Source: CAD feature listing. Evaluate the final solid. Frame: model axes, mm. Give positions to 0.01 mm unless a question says otherwise; leave off trailing zeros. Answer in a Markdown table with one row per item.
Autodesk Inventor part; units mm, degrees
ref_plane "YZ Plane" through (0, 0, 0) normal (1, 0, 0) x (0, 1, 0)
ref_plane "XZ Plane" through (0, 0, 0) normal (0, 1, 0) x (-1, 0, 0)
ref_plane "XY Plane" through (0, 0, 0) normal (0, 0, 1) x (1, 0, 0)
sketch "Sketch1" plane through (0, 0, 0) normal (1, 0, 0) x (0, 1, 0)
  line L0 (0, 0) -> (25.4, 0) construction
  line L1 (25.4, 0) -> (25.4, -1.5875) construction
  line L2 (25.4, -1.5875) -> (0, -1.5875) construction
  line L3 (0, -1.5875) -> (0, 0) construction
  circle A0 centre (4.7625, 3.175) radius 4.7625 construction
  line L4 (25.4, 0) -> (25.4, -1.5875)
  line L5 (25.4, -1.5875) -> (4.7625, -1.5875)
  line L6 (25.4, 0) -> (8.3123, 0)
  arc A1 (8.3123, 0) -> (4.7625, -1.5875) centre (4.7625, 3.175) ccw
  dimension "d0" = 25.4
  dimension "d1" = 1.5875
  dimension "d2" = 9.525
  dimension "d3" = 4.7625
  dimension "d4" = 3.175
extrude "Extrusion1" add sketch "Sketch1" along normal blind 635
sketch "Sketch2" plane through (635, 0, 0) normal (1, 0, 0) x (0, 0, -1)
  arc A0 (0, 8.3123) -> (1.5875, 4.7625) centre (-3.175, 4.7625) ccw
  circle A1 centre (-3.175, 4.7625) radius 3.175
  point P0 (0, 0)
  dimension "d7" = 6.35
extrude "Extrusion2" cut sketch "Sketch2" against normal blind 635
sketch "Sketch3" plane through (635, 0, 0) normal (1, 0, 0) x (0, 0, -1)
  circle A0 centre (-3.175, 4.7625) radius 3.175
  arc A1 (0, 8.3123) -> (1.5875, 4.7625) centre (-3.175, 4.7625) ccw
  line L0 (1.5875, 4.7625) -> (1.5875, 25.4)
  line L1 (0, 8.3123) -> (1.5875, 8.3123)
  line L2 (1.5875, 8.3123) -> (1.5875, 4.7625)
  arc A2 (0, 8.3123) -> (1.5875, 4.7625) centre (-3.175, 4.7625) ccw
  point P0 (0, 0)
extrude "Extrusion3" cut sketch "Sketch3" against normal blind 25.4
pattern_linear "Rectangular Pattern1" count 13 spacing 50.8 along (-1, 0, 0) of "Extrusion3"
sketch "Sketch4" plane through (635, 25.4, -1.5875) normal (0, 0, -1) x (-1, 0, 0)
  line L0 (635, 0) -> (0, 0)
  line L1 (0, -17.0877) -> (0, 0)
  point P0 (635, -25.4)
  point P1 (12.7, -9.525)
  dimension "d15" = 9.525
  dimension "d16" = 12.7
hole "Hole1" at (622.3, 15.875, -1.5875) direction (0, 0, 1) diameter 6.35 end through all
pattern_linear "Rectangular Pattern2" count 25 spacing 25.4 along (-1, 0, 0) of "Hole1"
properties part number "continuous hinge"
(1) Section query A-A (z = 3.75). Give the number of separate pieces and of enclosed holes in the cut face, plus the area to 3 significant figures.
A:
| item | result |
|---|---|
| separate pieces | 24 |
| enclosed holes | 0 |
| area | 979 mm^2 |
(2) Ray query, probe 1 along Y at (x, z) = (165.1, -1.1); probe 2 along Y at (x, z) = (596.9, -0.45); probe 3 along Z at (x, y) = (258.5, 10.25). Return the intervals inside material, ascending.
A:
| item | result |
|---|---|
| probe 1 | y = 8.31 to 12.7, 19.05 to 25.4 |
| probe 2 | y = 1.67 to 12.7, 19.05 to 25.4 |
| probe 3 | z = -1.59 to 0 |
(3) First-contact query: pin 1 Ø3 at (y, z) = (7, 5) entering from +X; pin 2 Ø1.3 at (x, z) = (312, -0.5) entering from -Y; pin 3 Ø4 at (x, z) = (541.5, 0.5) entering from +Y; pin 4 Ø8 at (x, y) = (144, 16.5) entering from +Z. Flat tips, straight axial feed; report the tip coordinate or a pass-through.
A:
| item | result |
|---|---|
| pin 1 | stops at x = 609.6 |
| pin 2 | stops at y = 8.31 |
| pin 3 | stops at y = 25.4 |
| pin 4 | stops at z = 0 |
